Verification items for the finished model (mm, model axes). A direction names the side the tool comes from. Coordinates: 2 decimals unless noted, no trailing zeros. Order: outer loops, then holes, each group sorted by start corner. A loop starts at its lowest first (then second) coordinate and runs counter-clockwise, first axis right, second up. Notation, with made-up numbers: M -15,-19.75 L 26,-19.75 A10 cw 26,-11.75 Z; hole C 21,74.5 d2. An arc over 180 degrees is marked long. Write item = value, one per line.
```python
from build123d import *

# Parameters (mm, degrees)
BOX_W     = 14
BOX_H     = 14
BOX_DEPTH = 14
FILLET_R  = 1


with BuildPart() as cone:
    # Cone → Cone (revolve)
    with BuildSketch(Plane(origin=(7, -5, 7), x_dir=(-1, 0, 0), z_dir=(0, 0, -1))):
        Polygon((0, 0), (2, 0), (4, 5), (0, 5), align=None)
    revolve(axis=Axis((7, -5, 7), (0, 1, 0)))


with BuildPart() as cone001:
    # Cone001 → Cone001 (revolve)
    with BuildSketch(Plane(origin=(19, 7, 7), x_dir=(0, -1, 0), z_dir=(0, 0, -1))):
        Polygon((0, 0), (2, 0), (4, 5), (0, 5), align=None)
    revolve(axis=Axis((19, 7, 7), (-1, 0, 0)))


with BuildPart() as cone002:
    # Cone002 → Cone002 (revolve)
    with BuildSketch(Plane(origin=(7, 19, 7), x_dir=(1, 0, 0), z_dir=(0, 0, -1))):
        Polygon((0, 0), (2, 0), (4, 5), (0, 5), align=None)
    revolve(axis=Axis((7, 19, 7), (0, -1, 0)))


with BuildPart() as cone003:
    # Cone003 → Cone003 (revolve)
    with BuildSketch(Plane(origin=(-5, 7, 7), x_dir=(0, 1, 0), z_dir=(0, 0, -1))):
        Polygon((0, 0), (2, 0), (4, 5), (0, 5), align=None)
    revolve(axis=Axis((-5, 7, 7), (1, 0, 0)))


with BuildPart() as fillet_body:
    # Box → Box (new body)
    with BuildSketch(Plane.XY):
        with Locations((7, 7)):
            Rectangle(BOX_W, BOX_H)
    extrude(amount=BOX_DEPTH)

    # Fillet
    fillet_edges = [fillet_body.edges().sort_by_distance(p)[0] for p in [
        (0, 0, 7),
        (0, 7, 14),
        (0, 14, 7),
        (14, 0, 7),
        (14, 7, 14),
        (14, 14, 7),
        (7, 0, 14),
        (7, 14, 14),
    ]]
    fillet(fillet_edges, radius=FILLET_R)


with BuildPart() as fusion:
    # Sphere → Sphere (revolve)
    with BuildSketch(Plane(origin=(7, 7, 20), x_dir=(1, 0, 0), z_dir=(0, -1, 0))):
        with BuildLine():
            ThreePointArc((0, -7), (7, 0), (0, 7))
            Line((0, 7), (0, -7))
        make_face()
    revolve(axis=Axis((7, 7, 20), (0, 0, 1)))

    # Fusion: union Cone, Cone001, Cone002, Cone003, Fillet body
    add(cone.part)
    add(cone001.part)
    add(cone002.part)
    add(cone003.part)
    add(fillet_body.part)


solid = fusion.part
```
Item 1: Gauge pin test, flat ends, axial feed: pin 1 (6 mm diameter, centred on y = 4, z = 6.5, fed in from -X); pin 2 (6 mm diameter, centred on x = 1, z = 17.5, fed in from +Y); pin 3 (1 mm diameter, centred on y = 4.5, z = 19, fed in from +X); pin 4 (6 mm diameter, centred on x = 5, y = 4.5, fed in from +Z). Record the tip position at first contact, or that the pin passes through.
Report:
pin_1 = -5
pin_2 = 13.06
pin_3 = 13.65
pin_4 = 27
Item 2: Sectioned sample at A-A, the plane z = 7. Enter the section's corners in (x, y), then the cut area to 3 significant figures.
Report:
outline = M -5,5 L 0,3 L 0,1 A1 ccw 1,0 L 3,0 L 5,-5 L 9,-5 L 11,0 L 13,0 A1 ccw 14,1 L 14,3 L 19,5 L 19,9 L 14,11 L 14,13 A1 ccw 13,14 L 11,14 L 9,19 L 5,19 L 3,14 L 1,14 A1 ccw 0,13 L 0,11 L -5,9 Z
area = 315 mm^2
Item 3: Release check for a two-part mould opening along Z. For faces 1 (the conical face through (17.576, 7.557, 4.492)), 2 (the flat face through (7, -5, 7)), 3 (the cylindrical face through (7.084, 13.715, 13.699)) record: pulls with the +Z half, pulls with the -Z half, needs draft (parallel to the pull), parting line crosses it, or undercut.
Report:
face_1 = parting line crosses it
face_2 = needs draft
face_3 = undercut
Item 4: Sectioned sample at C-C, the plane y = 7. Enter the section's corners in (x, z), then the cut area to 3 significant figures.
Report:
outline = M -5,5 L 0,3 L 0,0 L 14,0 L 14,3 L 19,5 L 19,9 L 14,11 L 14,13 A1 ccw 13,14 L 10.61,14 A7 ccw long 3.39,14 L 1,14 A1 ccw 0,13 L 0,11 L -5,9 Z
area = 405 mm^2
Item 5: Scan lines: L1, parallel to Z at x = 11.5, y = 5.5; L2, parallel to Y at x = 5, z = 3. Record each from-to range of solid material in increasing order. Write a range as from..to.
Report:
L1 = 0..14, 14.85..25.15
L2 = 0..14
Item 6: Tool access check on faces 4 (the flat face through (4, 0, 4)), 5 (the flat face through (14, 4, 4)), 6 (the flat face through (0, 4, 4)). Record the directions out of +Z, -Z, +X, -X, +Y, -Y that give a thin tool (end or side, any length) a straight path to the whole face; none if there is none.
Report:
face_4 = -Y
face_5 = +X
face_6 = -X
Item 7: Sectioned sample at B-B, the plane x = 11.5. Enter the section's corners in (y, z), then the cut area to 3 significant figures.
Report:
outline = M 0,0 L 14,0 L 14,13 A1 ccw 13,14 L 1,14 A1 ccw 0,13 Z; C 7,20 d10.72
area = 286 mm^2
